from build123d import *

# Parameters (mm, degrees)
SKETCH_1_R      = 10
SKETCH_1_R_2    = 3.26
SKETCH_1_R_3    = 1
EXTRUDE_1_DEPTH = 3
SKETCH_2_R      = 5
SKETCH_2_R_2    = 3.025
EXTRUDE_2_DEPTH = 2


with BuildPart() as part:
    # 草图1 → 凸台-拉伸1 (new body)
    with BuildSketch(Plane(origin=(0, 0, 0), x_dir=(1, 0, 0), z_dir=(0, 1, 0))):
        with Locations(Location((0, 0, 0), (0, 0, 270))):
            Circle(SKETCH_1_R)
        with Locations(Location((0, 0, 0), (0, 0, 270))):
            Circle(SKETCH_1_R_2, mode=Mode.SUBTRACT)
        with Locations(Location((0, 8, 0), (0, 0, 270))):
            Circle(SKETCH_1_R_3, mode=Mode.SUBTRACT)
        with Locations(Location((5.656854249, 5.656854249, 0), (0, 0, 270))):
            Circle(SKETCH_1_R_3, mode=Mode.SUBTRACT)
        with Locations(Location((8, 0, 0), (0, 0, 270))):
            Circle(SKETCH_1_R_3, mode=Mode.SUBTRACT)
        with Locations(Location((5.656854249, -5.656854249, 0), (0, 0, 270))):
            Circle(SKETCH_1_R_3, mode=Mode.SUBTRACT)
        with Locations(Location((0, -8, 0), (0, 0, 270))):
            Circle(SKETCH_1_R_3, mode=Mode.SUBTRACT)
        with Locations(Location((-5.656854249, -5.656854249, 0), (0, 0, 270))):
            Circle(SKETCH_1_R_3, mode=Mode.SUBTRACT)
        with Locations(Location((-8, 0, 0), (0, 0, 270))):
            Circle(SKETCH_1_R_3, mode=Mode.SUBTRACT)
        with Locations(Location((-5.656854249, 5.656854249, 0), (0, 0, 270))):
            Circle(SKETCH_1_R_3, mode=Mode.SUBTRACT)
    extrude(amount=EXTRUDE_1_DEPTH)

    # 草图2 → 凸台-拉伸2 (add)
    with BuildSketch(Plane(origin=(0, 3, 0), x_dir=(1, 0, 0), z_dir=(0, 1, 0))):
        with Locations(Location((0, 0, 0), (0, 0, 270))):
            Circle(SKETCH_2_R)
        with Locations(Location((0, 0, 0), (0, 0, 270))):
            Circle(SKETCH_2_R_2, mode=Mode.SUBTRACT)
    extrude(amount=EXTRUDE_2_DEPTH)


solid = part.part
Build history of the part. All positions in model axes, mm. A direction names the side the tool comes from. Give positions to 0.01 mm unless a question says otherwise; leave off trailing zeros. Order: outer loops, then holes, each group sorted by start corner. A loop starts at its lowest first (then second) coordinate and runs counter-clockwise, first axis right, second up. Notation, with made-up numbers: M 17.25,-3.5 L 31.25,-3.5 A18 cw 31.25,10.5 Z; hole C -9,82.25 d6. An arc over 180 degrees is marked long. Use one line per item in the form item = value.
1) Tool access for faces 4 (the face through (3.232, 1.479, -0.424)), 5 (the face through (9, 1, 0)), 6 (the face through (5, 3, 2)): list every direction of +Z, -Z, +X, -X, +Y, -Y with a clear straight run to the whole face (end or side of a thin tool).
Calculated:
face_4 = -Y
face_5 = +Y, -Y
face_6 = +Y
2) Saw through at B-B (x = 0). Give the cut face in (y, z) (3 decimals), plus the area to 3 significant figures.
Calculated:
outline = M 0,-10 L 3,-10 L 3,-9 L 0,-9 Z; M 0,-7 L 3,-7 L 3,-5 L 5,-5 L 5,-3.025 L 3,-3.025 L 3,-3.26 L 0,-3.26 Z; M 0,3.26 L 3,3.26 L 3,3.025 L 5,3.025 L 5,5 L 3,5 L 3,7 L 0,7 Z; M 0,9 L 3,9 L 3,10 L 0,10 Z
area = 36.3 mm2
3) Saw through at D-D (x = -8). Give the cut face in (y, z).
Calculated:
outline = M 0,-6 L 3,-6 L 3,-1 L 0,-1 Z; M 0,1 L 3,1 L 3,6 L 0,6 Z
4) Drop flat-ended pins along their axis: pin 1 (4 mm diameter, centred on x = 0.5, z = 1, fed in from -Y); pin 2 (2.5 mm diameter, centred on x = -5.66, z = -5.66, fed in from +Y); pin 3 (1 mm diameter, centred on x = -6.5, y = 2, fed in from +Z); pin 4 (1.8 mm diameter, centred on x = 5.66, z = 5.66, fed in from -Y). Give the stop position or say it passes through.
Calculated:
pin_1 = 3
pin_2 = 3
pin_3 = 8
pin_4 = through
5) Probe probe 1 along X at (y, z) = (4.5, 0) (3 decimals); probe 2 along Z at (x, y) = (-6.25, 2.6). List the from-to ranges inside material, lowest first.
Calculated:
probe_1 = -5 to -3.025, 3.025 to 5
probe_2 = -7.81 to -6.46, -4.85 to 4.85, 6.46 to 7.81
6) Saw through at C-C (z = 0). Give the cut face in (x, y) (3 decimals).
Calculated:
outline = M -10,0 L -9,0 L -9,3 L -10,3 Z; M -7,0 L -3.26,0 L -3.26,3 L -3.025,3 L -3.025,5 L -5,5 L -5,3 L -7,3 Z; M 3.025,3 L 3.26,3 L 3.26,0 L 7,0 L 7,3 L 5,3 L 5,5 L 3.025,5 Z; M 9,0 L 10,0 L 10,3 L 9,3 Z
7) Two-plate mould, pull along X, no slides. Class faces 1 (the face through (-4.665, 1.479, 5.527)), 2 (the face through (0, 0, 4)), 3 (the face through (-4.88, 3.99, -1.08)): released by +X, released by -X, zero draft, split by the parting line, or undercut.
Calculated:
face_1 = undercut
face_2 = zero draft
face_3 = split by the parting line
8) Saw through at A-A (z = -8). Give the cut face in (x, y).
Calculated:
outline = M -6,0 L -1,0 L -1,3 L -6,3 Z; M 1,0 L 6,0 L 6,3 L 1,3 Z
